Answer from the drawing. Dimensions are ordinates in mm from the lowest x, y and z of the part. A direction names the side the tool comes from. Coordinates: 2 decimals unless noted, no trailing zeros. Loops run counter-clockwise (first coordinate to the right, second up) from the corner with the lowest first, then second, coordinate; pieces in that order, holes last. Notation, with made-up numbers: M 54.25,65 L 97.25,65 A12 cw 97.25,84 Z; hole C 9.5,61.5 d2. An arc over 180 degrees is marked long. Answer as CSV lines item,"result". Start each with the question number.
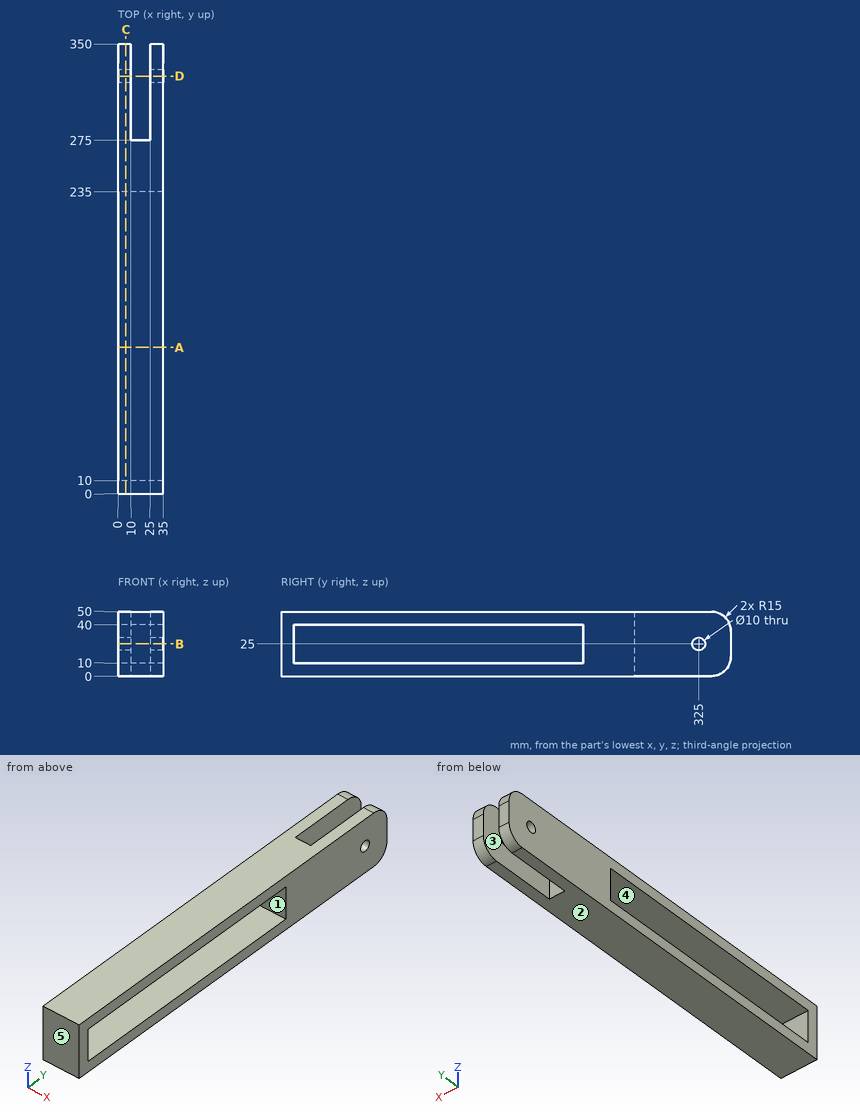
Item 1: Section C-C on x = 6 is taken. Determine the outline of the cut face in (y, z), then the cut area to 3 significant figures.
Item 2: Consider line 1 (Y direction, x = 28.25, z = 25); line 2 (Z direction, x = 4, y = 325); line 3 (X direction, y = 308, z = 45). Determine where each line is inside the solid, lowest interval first.
Item 3: Section D-D on y = 325 is taken. Determine the outline of the cut face in (x, z), then the cut area to 3 significant figures.
Item 4: For the marked faces 1 and 2, determine the directions among +Z, -Z, +X, -X, +Y, -Y from which every point of the face is accessible in a straight line to the end or side of a thin tool.
Item 5: Section B-B on z = 25 is taken. Determine the outline of the cut face in (x, y), then the cut area to 3 significant figures.
Item 6: Each of these flat-tipped pins is pushed along its axis until it touches: P1, Ø5, axis at x = 15, z = 25.5, coming from the +Y side; P2, Ø2, axis at x = 9, z = 20, coming from the -Y side. Where does it stop, or does it pass through?
Item 7: Section A-A on y = 114 is taken. Determine the outline of the cut face in (x, z), then the cut area to 3 significant figures.
Item 8: For a pull along Y with two mould halves and no side action, classify the marked faces 3, 4 and 5 as pulls with the +Y half, pulls with the -Y half, needs draft (parallel to the pull), parting line crosses it, or undercut.
Results are:
1,outline,"M 0,0 L 335,0 A15 ccw 350,15 L 350,35 A15 ccw 335,50 L 0,50 Z; hole M 10,10 L 235,10 L 235,40 L 10,40 Z; hole C 325,25 d10"
1,area,"10,600 mm²"
2,line 1,"0 to 10, 235 to 320, 330 to 350"
2,line 2,"0 to 20, 30 to 50"
2,line 3,"0 to 10, 25 to 35"
3,outline,"M 0,0 L 10,0 L 10,20 L 0,20 Z; M 0,30 L 10,30 L 10,50 L 0,50 Z; M 25,0 L 35,0 L 35,20 L 25,20 Z; M 25,30 L 35,30 L 35,50 L 25,50 Z"
3,area,"800 mm²"
4,face 1,"+X, -X"
4,face 2,"-Z, +X, -X, +Y, -Y"
5,outline,"M 0,0 L 35,0 L 35,10 L 0,10 Z; M 0,235 L 35,235 L 35,320 L 25,320 L 25,275 L 10,275 L 10,320 L 0,320 Z; M 0,330 L 10,330 L 10,350 L 0,350 Z; M 25,330 L 35,330 L 35,350 L 25,350 Z"
5,area,"3,050 mm²"
6,P1,"y = 275"
6,P2,"y = 0"
7,outline,"M 0,0 L 35,0 L 35,10 L 0,10 Z; M 0,40 L 35,40 L 35,50 L 0,50 Z"
7,area,"700 mm²"
8,face 3,"needs draft"
8,face 4,"undercut"
8,face 5,"pulls with the -Y half"
